Design review of the part built by this model. Coordinates are the model's own, in mm. A direction names the side the tool comes from. Round coordinates to 2 decimals unless told otherwise and drop trailing zeros. Order: outer loops, then holes, each group sorted by start corner. A loop starts at its lowest first (then second) coordinate and runs counter-clockwise, first axis right, second up. Notation, with made-up numbers: (23.5, -39) - (62.5, -39) arc R13 ccw to (62.5, -29) - close; hole circle Ø1 at (86.25, 15.25). An arc over 180 degrees is marked (long way). Write item = value, one per line.
from build123d import *

# Parameters (mm, degrees)
SKETCH1_R           = 60
BOSS_EXTRUDE1_DEPTH = 15
SKETCH3_W           = 30
SKETCH3_H           = 30
BOSS_EXTRUDE2_DEPTH = 170
SKETCH4_W           = 20
SKETCH4_H           = 40
CUT_EXTRUDE1_DEPTH  = 20


with BuildPart() as part:
    # Sketch1 → Boss-Extrude1 (new body)
    with BuildSketch(Plane(origin=(0, 0, 0), x_dir=(1, 0, 0), z_dir=(0, 1, 0))):
        Circle(SKETCH1_R)
    extrude(amount=BOSS_EXTRUDE1_DEPTH)

    # Sketch3 → Boss-Extrude2 (add)
    with BuildSketch(Plane(origin=(0, 15, 0), x_dir=(1, 0, 0), z_dir=(0, 1, 0))):
        Rectangle(SKETCH3_W, SKETCH3_H)
    extrude(amount=BOSS_EXTRUDE2_DEPTH)

    # Sketch4 → Cut-Extrude1 (cut)
    with BuildSketch(Plane.XY.offset(15)):
        with Locations((0, 160)):
            Rectangle(SKETCH4_W, SKETCH4_H)
    extrude(amount=-CUT_EXTRUDE1_DEPTH, mode=Mode.SUBTRACT)


solid = part.part
1) For faces 1 (the flat face through (0, 185, 0)), 2 (the flat face through (-10, 160, 5)), 3 (the flat face through (0, 80, 15)), list the 3-axis set-ups (+Z, -Z, +X, -X, +Y, -Y) from which the entire face can be reached by the end or side of a thin tool; tool diameter is ignored.
Findings:
face_1 = +Z, -Z, +X, -X, +Y
face_2 = +Z
face_3 = +Z, +X, -X, +Y
2) We need section A-A on z = 0. Write out the cut boundary in (x, y).
Findings:
outline = (-60, 0) - (60, 0) - (60, 15) - (15, 15) - (15, 185) - (-15, 185) - (-15, 15) - (-60, 15) - close; hole (-10, 140) - (10, 140) - (10, 180) - (-10, 180) - close
3) Clearance check with flat-ended pins moving along their axes: pin 1 Ø10 at (y, z) = (166.5, 7) entering from +X; pin 2 Ø15 at (y, z) = (110, 4) entering from -X; pin 3 Ø3 at (y, z) = (88, 18) entering from -X; pin 4 Ø10 at (x, y) = (-4, 165.5) entering from +Z. State where each tip first meets the part, or that it passes through.
Findings:
pin_1 = 15
pin_2 = -15
pin_3 = through
pin_4 = -5
4) We need section C-C on y = 83. Write out the cut boundary in (x, z), and give its area (3 significant figures).
Findings:
outline = (-15, -15) - (15, -15) - (15, 15) - (-15, 15) - close
area = 900 mm^2
5) To check wall thickness, follow L1, parallel to Y at x = 53, z = -11.5; L2, parallel to Z at x = -3.5, y = 45; L3, parallel to Z at x = 6, y = 151.5. State the ranges of each line that lie inside material, in increasing order. Write a range as from..to.
Findings:
L1 = 0..15
L2 = -15..15
L3 = -15..-5
6) The part is to be moulded in two halves that separate along X. For faces 4 (the flat face through (0, 99, -15)), 5 (the flat face through (0, 160, -5)), 6 (the flat face through (-15, 99, 0)), 7 (the flat face through (15, 99, 0)), say which applies: released by +X, released by -X, zero draft, split by the parting line, or undercut.
Findings:
face_4 = zero draft
face_5 = undercut
face_6 = released by -X
face_7 = released by +X
7) We need section B-B on x = 0. Write out the cut boundary in (y, z), and give its area (3 significant figures).
Findings:
outline = (0, -60) - (15, -60) - (15, -15) - (185, -15) - (185, 15) - (180, 15) - (180, -5) - (140, -5) - (140, 15) - (15, 15) - (15, 60) - (0, 60) - close
area = 6,100 mm^2
8) We need section D-D on z = 36.5. Write out the cut boundary in (x, y), and give its area (3 significant figures).
Findings:
outline = (-47.62, 0) - (47.62, 0) - (47.62, 15) - (-47.62, 15) - close
area = 1,430 mm^2
